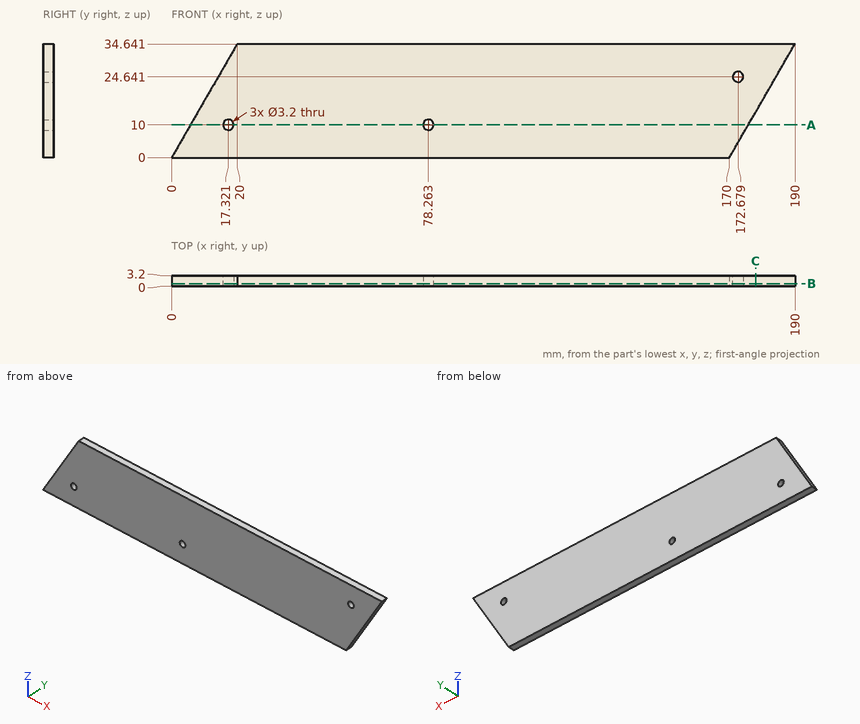
Design review of the part shown in the three views and the two pictorial views. Dimensions are in mm from the part's minimum x, y and z. Give positions to 0.01 mm unless a question says otherwise; leave off trailing zeros. Order: outer loops, then holes, each group sorted by start corner. A loop starts at its lowest first (then second) coordinate and runs counter-clockwise, first axis right, second up. Notation, with made-up numbers: M 2.5,64.5 L 36.5,64.5 A24 cw 36.5,80.5 Z; hole C -25,-2 d3. An arc over 180 degrees is marked long. Answer in a Markdown table with one row per item. Add a question column.
(1) Consider section B-B on y = 0.8. State the section outline as (x, z) points.
(2) Consider section A-A on z = 10. State the section outline as (x, y) points.
(3) Wall thickness on probe 1 along X at (y, z) = (2.1, 26) (1 decimal); probe 2 along Z at (x, y) = (174, 1.45) (1 decimal); probe 3 along X at (y, z) = (1.5, 3.5): over which ranges is each line inside the solid? List them lowest first. Write a range as [from, to].
(4) Consider section C-C on x = 178. State the section outline as (y, z) points.
Evaluation:
| question | item | result |
|---|---|---|
| 1 | outline | M 0,0 L 170,0 L 190,34.64 L 20,34.64 Z; hole C 17.32,10 d3.2; hole C 78.26,10 d3.2; hole C 172.68,24.64 d3.2 |
| 2 | outline | M 5.77,0 L 15.72,0 L 15.72,3.2 L 5.77,3.2 Z; M 18.92,0 L 76.66,0 L 76.66,3.2 L 18.92,3.2 Z; M 79.86,0 L 175.77,0 L 175.77,3.2 L 79.86,3.2 Z |
| 3 | probe 1 | x = [15, 171.8], [173.5, 185] |
| 3 | probe 2 | z = [6.9, 23.7], [25.5, 34.6] |
| 3 | probe 3 | x = [2.02, 172.02] |
| 4 | outline | M 0,13.86 L 3.2,13.86 L 3.2,34.64 L 0,34.64 Z |
